Work out the finished part from the listing and answer in its coordinate system (mm). A direction names the side the tool comes from. Round coordinates to 2 decimals unless told otherwise and drop trailing zeros. Loops run counter-clockwise (first coordinate to the right, second up) from the corner with the lowest first, then second, coordinate; pieces in that order, holes last. Notation, with made-up numbers: (52.25, 28.25) -> (64.25, 28.25) arc R25 ccw to (64.25, 43.25) -> close; hole circle Ø5 at (75, -8.5). An arc over 180 degrees is marked (long way). Use one line per item in the form item = value.
```python
from build123d import *

# Parameters (mm, degrees)
RESSALTO_EXTRUS_O1_DEPTH = 36
ESBO_O2_R                = 6
CORTE_EXTRUS_O1_DEPTH    = 37
ESBO_O4_R                = 2.5
CORTE_EXTRUS_O2_DEPTH    = 29


with BuildPart() as part:
    # Esboço1 → Ressalto-extrusão1 (new body)
    with BuildSketch(Plane.XY):
        Polygon((6.3777561, -6.012123693), (-6.3777561, -6.012123693), (-11.089070113, -2.012123693), (-19.410929887, -2.012123693), (-19.410929887, 12.63872394), (-21, 13.987876307), (-21, 21.987876307), (21, 21.987876307), (21, 13.987876307), (19.410929887, 12.63872394), (19.410929887, -2.012123693), (11.089070113, -2.012123693), align=None)
    extrude(amount=RESSALTO_EXTRUS_O1_DEPTH)

    # Esboço2 → Corte-extrusão1 (cut, through all)
    with BuildSketch(Plane.XY.offset(36)):
        with Locations((0, 6.987876307)):
            Circle(ESBO_O2_R)
    extrude(amount=-CORTE_EXTRUS_O1_DEPTH, mode=Mode.SUBTRACT)

    # Esboço4 → Corte-extrusão2 (cut, through all)
    with BuildSketch(Plane.XZ.offset(6.012123693)):
        with Locations((-15.25, 5)):
            Circle(ESBO_O4_R)
        with Locations((-15.25, 31)):
            Circle(ESBO_O4_R)
        with Locations((15.25, 5)):
            Circle(ESBO_O4_R)
        with Locations((15.25, 31)):
            Circle(ESBO_O4_R)
    extrude(amount=-CORTE_EXTRUS_O2_DEPTH, mode=Mode.SUBTRACT)


solid = part.part
```
(1) For a pull along Z with two mould halves and no side action, classify faces 1 (the flat face through (0, 14, 36)), 2 (the cylindrical face through (-17.09, 9.82, 6.69)), 3 (the cylindrical face through (-4.761, 3.337, 18.252)) as +Z half, -Z half, draft (parallel to the pull), parting line (faces both ways), or undercut.
Completed:
face_1 = +Z half
face_2 = undercut
face_3 = draft
(2) Consider L1, parallel to Z at x = -15.25, y = 14.5; L2, parallel to X at y = 14.75, z = 29.5; L3, parallel to X at y = 19.25, z = 4.5. Determine where each line is inside the solid, lowest interval first.
Completed:
L1 = 0 to 2.5, 7.5 to 28.5, 33.5 to 36
L2 = -21 to -17.25, -13.25 to 13.25, 17.25 to 21
L3 = -21 to -17.7, -12.8 to 12.8, 17.7 to 21
(3) Find section A-A, the plane x = 15.25. Write down the section's boundary in (y, z).
Completed:
outline = (-2.01, 0) -> (21.99, 0) -> (21.99, 2.5) -> (-2.01, 2.5) -> close; (-2.01, 7.5) -> (21.99, 7.5) -> (21.99, 28.5) -> (-2.01, 28.5) -> close; (-2.01, 33.5) -> (21.99, 33.5) -> (21.99, 36) -> (-2.01, 36) -> close
(4) Find section C-C, the plane y = 3.25. Write down the section's boundary in (x, z), then the cut area to 3 significant figures.
Completed:
outline = (-19.41, 0) -> (-4.69, 0) -> (-4.69, 36) -> (-19.41, 36) -> close; (4.69, 0) -> (19.41, 0) -> (19.41, 36) -> (4.69, 36) -> close; hole circle Ø5 at (-15.25, 5); hole circle Ø5 at (-15.25, 31); hole circle Ø5 at (15.25, 5); hole circle Ø5 at (15.25, 31)
area = 981 mm2
(5) For faces 4 (the flat face through (-15, -2.012, 18)), 5 (the cylindrical face through (12.752, 9.82, 5.11)), 6 (the flat face through (15, -2.012, 18)), determine the directions among +Z, -Z, +X, -X, +Y, -Y from which every point of the face is accessible in a straight line to the end or side of a thin tool.
Completed:
face_4 = +Z, -Z, -X, -Y
face_5 = +Y, -Y
face_6 = +Z, -Z, +X, -Y
(6) Given P1, Ø6, axis at x = 15.5, z = 7.5, coming from the -Y side; P2, Ø6, axis at y = 4.5, z = 30, coming from the -X side; P3, Ø8, axis at x = -15.25, z = 31, coming from the +Y side; P4, Ø2, axis at y = 2, z = 21.5, coming from the +X side, each flat-ended and moving along its own axis, determine where each tip first touches the part or whether it passes through.
Completed:
P1 = -2.01
P2 = -19.41
P3 = 21.99
P4 = 19.41
(7) Find section B-B, the plane z = 5. Write down the section's boundary in (x, y), then the cut area to 3 significant figures.
Completed:
outline = (-21, 13.99) -> (-19.41, 12.64) -> (-19.41, -2.01) -> (-17.75, -2.01) -> (-17.75, 21.99) -> (-21, 21.99) -> close; (-12.75, -2.01) -> (-11.09, -2.01) -> (-6.38, -6.01) -> (6.38, -6.01) -> (11.09, -2.01) -> (12.75, -2.01) -> (12.75, 21.99) -> (-12.75, 21.99) -> close; (17.75, -2.01) -> (19.41, -2.01) -> (19.41, 12.64) -> (21, 13.99) -> (21, 21.99) -> (17.75, 21.99) -> close; hole circle Ø12 at (0, 6.99)
area = 676 mm2
(8) Find section D-D, the plane x = 0. Write down the section's boundary in (y, z).
Completed:
outline = (-6.01, 0) -> (0.99, 0) -> (0.99, 36) -> (-6.01, 36) -> close; (12.99, 0) -> (21.99, 0) -> (21.99, 36) -> (12.99, 36) -> close
